Autodesk Inventor part; units mm, degrees
ref_plane "YZ Plane" through (0, 0, 0) normal (1, 0, 0) x (0, 1, 0)
ref_plane "XZ Plane" through (0, 0, 0) normal (0, 1, 0) x (-1, 0, 0)
ref_plane "XY Plane" through (0, 0, 0) normal (0, 0, 1) x (1, 0, 0)
sketch "Sketch1" plane through (0, 0, 0) normal (0, 1, 0) x (-1, 0, 0)
  circle A0 centre (368.3, 203.2) radius 2.54
  circle A1 centre (368.3, 241.3) radius 3.302
  circle A2 centre (368.3, 127) radius 2.54
  circle A3 centre (368.3, 88.9) radius 3.302
  circle A4 centre (368.3, 50.8) radius 2.54
  circle A5 centre (368.3, 12.7) radius 3.302
  line L0 (190.5, 244.602) -> (330.2, 244.602)
  line L1 (330.2, 244.602) -> (190.5, 244.602)
  arc A6 (330.2, 237.998) -> (330.2, 244.602) centre (330.2, 241.3) ccw
  line L2 (190.5, 237.998) -> (330.2, 237.998)
  line L3 (381, 251.46) -> (381, 2.54)
  line L4 (378.46, 0) -> (355.6, 0)
  line L5 (355.6, 0) -> (355.6, 0)
  circle A7 centre (368.3, 38.1) radius 2.54
  circle A8 centre (368.3, 63.5) radius 2.54
  circle A9 centre (368.3, 127) radius 2.54
  circle A10 centre (368.3, 114.3) radius 2.54
  circle A11 centre (368.3, 139.7) radius 2.54
  circle A12 centre (368.3, 203.2) radius 2.54
  circle A13 centre (368.3, 190.5) radius 2.54
  circle A14 centre (368.3, 215.9) radius 2.54
  line L6 (355.6, 0) -> (355.6, 25.4) construction
  line L7 (355.6, 25.4) -> (381, 25.4) construction
  line L8 (368.3, 88.9) -> (355.6, 88.9) construction
  arc A15 (352.298, 76.2) -> (358.902, 76.2) centre (355.6, 76.2) ccw
  arc A16 (358.902, 101.6) -> (352.298, 101.6) centre (355.6, 101.6) ccw
  line L9 (358.902, 76.2) -> (358.902, 101.6)
  line L10 (352.298, 101.6) -> (352.298, 76.2)
  line L11 (368.3, 139.7) -> (368.3, 165.1) construction
  line L12 (368.3, 165.1) -> (355.6, 165.1) construction
  arc A17 (352.298, 152.4) -> (358.902, 152.4) centre (355.6, 152.4) ccw
  arc A18 (358.902, 177.8) -> (352.298, 177.8) centre (355.6, 177.8) ccw
  line L13 (358.902, 152.4) -> (358.902, 177.8)
  line L14 (352.298, 177.8) -> (352.298, 152.4)
  arc A19 (342.9, 12.7) -> (355.6, 0) centre (355.6, 12.7) ccw
  line L15 (378.46, 254) -> (190.5, 254)
  arc A20 (378.46, 0) -> (381, 2.54) centre (378.46, 2.54) ccw
  arc A21 (381, 251.46) -> (378.46, 254) centre (378.46, 251.46) ccw
  line L16 (190.5, 228.6) -> (190.5, 159.7209) construction
  line L17 (330.2, 215.9) -> (190.5, 215.9)
  line L18 (342.9, 12.7) -> (342.9, 203.2)
  arc A22 (342.9, 203.2) -> (330.2, 215.9) centre (330.2, 203.2) ccw
  circle A23 centre (12.7, 203.2) radius 2.54
  circle A24 centre (12.7, 241.3) radius 3.302
  circle A25 centre (12.7, 127) radius 2.54
  circle A26 centre (12.7, 88.9) radius 3.302
  circle A27 centre (12.7, 50.8) radius 2.54
  circle A28 centre (12.7, 12.7) radius 3.302
  line L19 (190.5, 244.602) -> (50.8, 244.602)
  line L20 (50.8, 244.602) -> (190.5, 244.602)
  arc A29 (50.8, 244.602) -> (50.8, 237.998) centre (50.8, 241.3) ccw
  line L21 (190.5, 237.998) -> (50.8, 237.998)
  line L22 (0, 251.46) -> (0, 2.54)
  line L23 (2.54, 0) -> (25.4, 0)
  line L24 (25.4, 0) -> (25.4, 0)
  circle A30 centre (12.7, 38.1) radius 2.54
  circle A31 centre (12.7, 63.5) radius 2.54
  circle A32 centre (12.7, 139.7) radius 2.54
  circle A33 centre (12.7, 127) radius 2.54
  circle A34 centre (12.7, 114.3) radius 2.54
  circle A35 centre (12.7, 215.9) radius 2.54
  circle A36 centre (12.7, 203.2) radius 2.54
  circle A37 centre (12.7, 190.5) radius 2.54
  line L25 (25.4, 0) -> (25.4, 25.4) construction
  line L26 (25.4, 25.4) -> (0, 25.4) construction
  line L27 (12.7, 88.9) -> (25.4, 88.9) construction
  arc A38 (22.098, 76.2) -> (28.702, 76.2) centre (25.4, 76.2) ccw
  arc A39 (28.702, 101.6) -> (22.098, 101.6) centre (25.4, 101.6) ccw
  line L28 (22.098, 76.2) -> (22.098, 101.6)
  line L29 (28.702, 101.6) -> (28.702, 76.2)
  line L30 (12.7, 139.7) -> (12.7, 165.1) construction
  line L31 (12.7, 165.1) -> (25.4, 165.1) construction
  line L32 (22.098, 152.4) -> (22.098, 177.8)
  arc A40 (22.098, 152.4) -> (28.702, 152.4) centre (25.4, 152.4) ccw
  line L33 (28.702, 177.8) -> (28.702, 152.4)
  arc A41 (28.702, 177.8) -> (22.098, 177.8) centre (25.4, 177.8) ccw
  arc A42 (25.4, 0) -> (38.1, 12.7) centre (25.4, 12.7) ccw
  line L34 (2.54, 254) -> (190.5, 254)
  arc A43 (0, 2.54) -> (2.54, 0) centre (2.54, 2.54) ccw
  arc A44 (2.54, 254) -> (0, 251.46) centre (2.54, 251.46) ccw
  line L35 (50.8, 215.9) -> (190.5, 215.9)
  line L36 (38.1, 12.7) -> (38.1, 203.2)
  arc A45 (50.8, 215.9) -> (38.1, 203.2) centre (50.8, 203.2) ccw
  point P0 (381, 254)
  point P1 (381, 0)
  point P2 (342.9, 0)
  point P3 (342.9, 228.6)
  point P4 (0, 254)
  point P5 (0, 0)
  point P6 (38.1, 0)
  point P7 (38.1, 228.6)
  dimension "d2" = 12.7
  dimension "d3" = 228.6
  dimension "d6" = 25.4
  dimension "d7" = 25.4
  dimension "d8" = 12.7
  dimension "d10" = 25.4
  dimension "d12" = 12.7
  dimension "d17" = 12.7
extrude "Extrusion3" add sketch "Sketch1" along normal blind 6.35
properties part number "vrRig_v08p1_base"
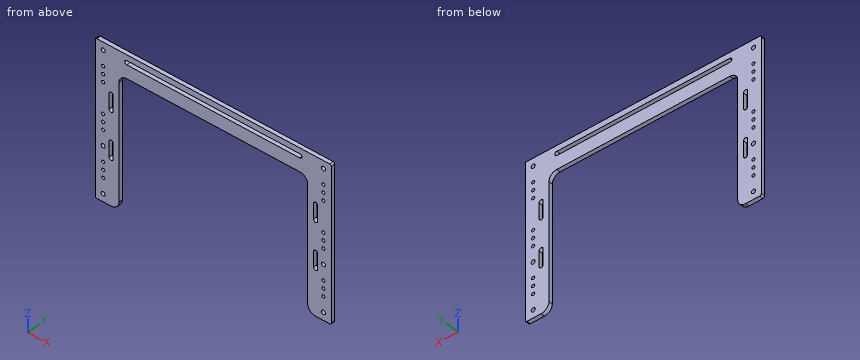
Design review of the part built by this model. Coordinates are the model's own, in mm. Coordinates: 2 decimals unless noted, no trailing zeros. Loops run counter-clockwise (first coordinate to the right, second up) from the corner with the lowest first, then second, coordinate; pieces in that order, holes last. Notation, with made-up numbers: (13, -25.5) - (29, -25.5) arc R22 ccw to (29, 12.5) - close; hole circle Ø10 at (44.5, 74.5). An arc over 180 degrees is marked (long way). Use CSV: the item, a comma, the result in double quotes. Start each with the question number.
1. Add section B-B on z = 166. Give the boundary of the cut face in (x, y).
2. Add section C-C on y = 1.25. Count the separate pieces of the cut face and the enclosed holes in it, plus the area to 3 significant figures.
3. Clearance check with a flat-ended pin moving along its axis: pin 1 (6 mm diameter, centred on x = -12.7, z = 203.2, fed in from +Y). State where the tip first meets the part, or that it passes through.
4. To check wall thickness, follow probe 1 along Z at (x, y) = (-163, 2.5); probe 2 along X at (y, z) = (5.5, 112.5); probe 3 along X at (y, z) = (0.75, 218). State the ranges of each line that lie inside material, in increasing order.
5. Add section A-A on x = -174. Give the boundary of the cut face in (y, z), plus the area to 3 significant figures.
Resolved:
1,outline,"(-381, 0) - (-358.9, 0) - (-358.9, 6.35) - (-381, 6.35) - close; (-352.3, 0) - (-342.9, 0) - (-342.9, 6.35) - (-352.3, 6.35) - close; (-38.1, 0) - (-28.7, 0) - (-28.7, 6.35) - (-38.1, 6.35) - close; (-22.1, 0) - (0, 0) - (0, 6.35) - (-22.1, 6.35) - close"
2,separate pieces,"1"
2,enclosed holes,"29"
2,area,"27,700 mm2"
3,pin 1,"y = 6.35"
4,probe 1,"215.9 to 238, 244.6 to 254"
4,probe 2,"-381 to -370.09, -366.51 to -342.9, -38.1 to -14.49, -10.91 to 0"
4,probe 3,"-381 to -369.73, -366.87 to -14.13, -11.27 to 0"
5,outline,"(0, 215.9) - (6.35, 215.9) - (6.35, 238) - (0, 238) - close; (0, 244.6) - (6.35, 244.6) - (6.35, 254) - (0, 254) - close"
5,area,"200 mm2"
